```python
from build123d import *

# Parameters (mm, degrees)
F0_R           = 1.5
F1_DEPTH       = 6
F3_DEPTH       = 21
F5_D           = 2.7
F5_DEPTH       = 9.5
F5_CSINK_D     = 3
F5_CSINK_ANGLE = 90
F5_TIP         = 0.8111618357
F8_SIZE        = 0.5


with BuildPart() as f1:
    # F0 (on Top) → F1 (new body)
    with BuildSketch(Plane.XY):
        Circle(F0_R)
    extrude(amount=F1_DEPTH)

    # F2 (on face) → F3 (join)
    with BuildSketch(Plane.XY.offset(6)):
        Polygon((-1.443375673, -2.5), (1.443375673, -2.5), (2.8867513459, 0), (1.443375673, 2.5), (-1.443375673, 2.5), (-2.8867513459, 0), align=None)
    extrude(amount=F3_DEPTH)

    # F5
    with Locations(Plane.XY.offset(27)):
        with Locations((0, 0)):
            CounterSinkHole(F5_D / 2, F5_CSINK_D / 2, depth=F5_DEPTH, counter_sink_angle=F5_CSINK_ANGLE)
            with Locations((0, 0, -(F5_DEPTH + F5_TIP / 2))):  # 118° drill point
                Cone(0, F5_D / 2, F5_TIP, mode=Mode.SUBTRACT)

    # F6 (on Front) → F7 (revolve, cut)
    with BuildSketch(Plane.XZ):
        Polygon((-3.6906760422, 6.4588518128), (-3.6906760422, 6), (-2.5, 6), align=None)
        Polygon((-3.6226674233, 26.5411481872), (-2.4319913811, 27), (-3.6226674233, 27), align=None)
    revolve(axis=Axis((0, 0, 14.2609653992), (0, 0, 1)), mode=Mode.SUBTRACT)

    # F8
    f8_edges = [f1.edges().sort_by_distance(p)[0] for p in [
        (-1.5, 0, 0),
    ]]
    chamfer(f8_edges, length=F8_SIZE)


solid = f1.part
```
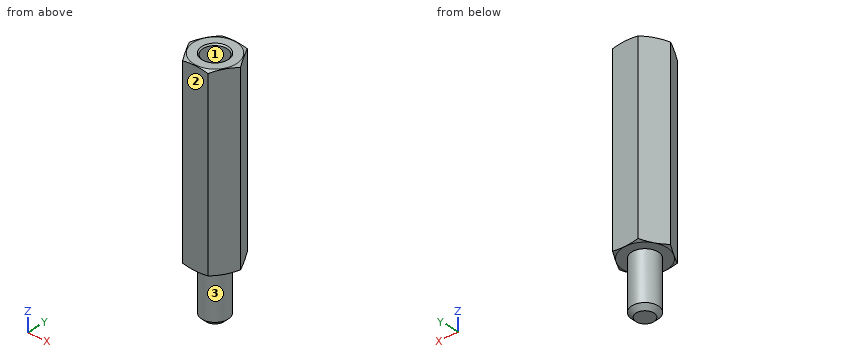
Design review of the part built by this model. Coordinates are the model's own, in mm. Face numbers are marked on the shaded views. A direction names the side the tool comes from. Give positions to 0.01 mm unless a question says otherwise; leave off trailing zeros. Order: outer loops, then holes, each group sorted by start corner. A loop starts at its lowest first (then second) coordinate and runs counter-clockwise, first axis right, second up. Notation, with made-up numbers: (-14, 20) -> (20, 20) arc R9 ccw to (20, 29) -> close; hole circle Ø7 at (6, 78). An arc over 180 degrees is marked (long way). Write item = value, one per line. Start each with the question number.
(1) We need section B-B on z = 10.25. Write out the cut boundary in (x, y), plus the area to 3 significant figures.
(2) We need section A-A on z = 19.5. Write out the cut boundary in (x, y), plus the area to 3 significant figures.
(3) To check wall thickness, follow line 1 along Y through (x, z) = (0, 24.5); line 2 along Z through (x, y) = (1.5, -0.3); line 3 along Y through (x, z) = (2.6, 25). State the ranges of each line that lie inside material, in increasing order.
(4) We need section C-C on z = 1.75. Write out the cut boundary in (x, y).
(5) For the marked faces 1, 2 and 3, list the 3-axis set-ups (+Z, -Z, +X, -X, +Y, -Y) from which the entire face can be reached by the end or side of a thin tool; tool diameter is ignored.
Numbers:
q1.outline = (-2.89, 0) -> (-1.44, -2.5) -> (1.44, -2.5) -> (2.89, 0) -> (1.44, 2.5) -> (-1.44, 2.5) -> close
q1.area = 21.7 mm^2
q2.outline = (-2.89, 0) -> (-1.44, -2.5) -> (1.44, -2.5) -> (2.89, 0) -> (1.44, 2.5) -> (-1.44, 2.5) -> close; hole circle Ø2.7 at (0, 0)
q2.area = 15.9 mm^2
q3.line_1 = -2.5 to -1.35, 1.35 to 2.5
q3.line_2 = 6 to 27
q3.line_3 = -0.5 to 0.5
q4.outline = circle Ø3 at (0, 0)
q5.face_1 = +Z
q5.face_2 = +Z, -Z, +X, -X, -Y
q5.face_3 = -Z
